from build123d import *

# Parameters (mm, degrees)
RESSALTO_EXTRUS_O1_DEPTH = 160
FILETE1_R                = 0.5
ESBO_O2_R                = 1.5
CORTE_EXTRUS_O1_DEPTH    = 161


with BuildPart() as part:
    # Esboço1 → Ressalto-extrusão1 (new body)
    with BuildSketch(Plane(origin=(0, 0, 0), x_dir=(-1, 0, 0), z_dir=(0, 0, -1))):
        Polygon((67.502122675, -1.443375673), (70.002122675, -2.886751346), (72.502122675, -1.443375673), (72.502122675, 1.443375673), (70.002122675, 2.886751346), (67.502122675, 1.443375673), align=None)
    extrude(amount=-RESSALTO_EXTRUS_O1_DEPTH)

    # Filete1
    filete1_edges = [part.edges().sort_by_distance(p)[0] for p in [
        (-71.252122675, -2.165063509, 160),
        (-72.502122675, 0, 160),
        (-71.252122675, 2.165063509, 160),
        (-68.752122675, 2.165063509, 160),
        (-67.502122675, 0, 160),
        (-68.752122675, 2.165063509, 0),
        (-71.252122675, 2.165063509, 0),
        (-72.502122675, 0, 0),
        (-71.252122675, -2.165063509, 0),
        (-68.752122675, -2.165063509, 0),
        (-67.502122675, 0, 0),
        (-68.752122675, -2.165063509, 160),
    ]]
    fillet(filete1_edges, radius=FILETE1_R)

    # Esboço2 → Corte-extrusão1 (cut, through all)
    with BuildSketch(Plane.XY.offset(160)):
        with Locations((-70.002122675, 0)):
            Circle(ESBO_O2_R)
    extrude(amount=-CORTE_EXTRUS_O1_DEPTH, mode=Mode.SUBTRACT)


solid = part.part
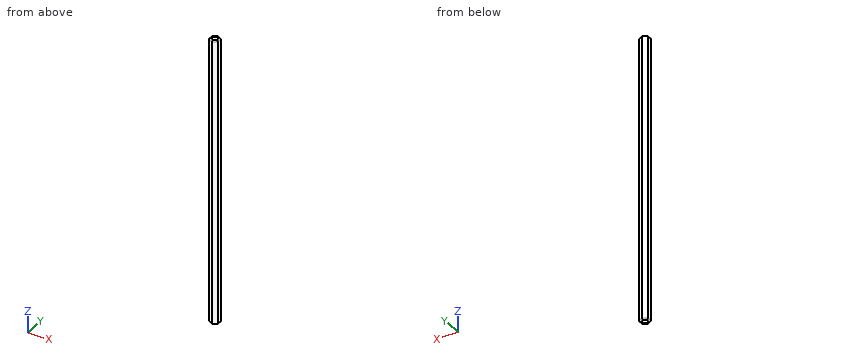
Work out the finished part from the listing and answer in its coordinate system (mm). Coordinates: 2 decimals unless noted, no trailing zeros. Loops run counter-clockwise (first coordinate to the right, second up) from the corner with the lowest first, then second, coordinate; pieces in that order, holes last. Notation, with made-up numbers: M -34,74 L -18,74 A16 ccw -18,88 Z; hole C 31,15.5 d2. An arc over 180 degrees is marked long. Answer in a Markdown table with one row per item. Add a question column.
1. Consider L1, parallel to X at y = 0.1, z = 9; L2, parallel to Y at x = -68.95, z = 107; L3, parallel to X at y = -0.65, z = 119. Determine where each line is inside the solid, lowest interval first.
2. A flat-ended cylindrical pin translates along its axis: P1, Ø2, axis at x = -71, y = 2, coming from the -Z side. Find the tip coordinate at first contact, or state that the pin passes through.
3. Find section B-B, the plane z = 143. Write down the section's boundary in (x, y).
4. Find section A-A, the plane y = 0. Write down the section's boundary in (x, z).
Reported:
| question | item | result |
|---|---|---|
| 1 | L1 | x = -72.5 to -71.5, -68.51 to -67.5 |
| 1 | L2 | y = -2.28 to -1.07, 1.07 to 2.28 |
| 1 | L3 | x = -72.5 to -71.35, -68.65 to -67.5 |
| 2 | P1 | stops at z = 0 |
| 3 | outline | M -72.5,-1.44 L -70,-2.89 L -67.5,-1.44 L -67.5,1.44 L -70,2.89 L -72.5,1.44 Z; hole C -70,0 d3 |
| 4 | outline | M -72.5,0.5 A0.5 ccw -72,0 L -71.5,0 L -71.5,160 L -72,160 A0.5 ccw -72.5,159.5 Z; M -68.5,0 L -68,0 A0.5 ccw -67.5,0.5 L -67.5,159.5 A0.5 ccw -68,160 L -68.5,160 Z |
